Input: part model. Units: mm. Frame: model coordinates. A direction names the side the tool comes from. Round coordinates to 2 decimals unless told otherwise and drop trailing zeros. Loops run counter-clockwise (first coordinate to the right, second up) from the corner with the lowest first, then second, coordinate; pieces in that order, holes last.
1) Ray query, line 1 along Y through (x, z) = (-5, 1.45); line 2 along X through (y, z) = (-1.75, 1.5); line 3 along X through (y, z) = (4.5, 1.05). Return the intervals inside material, ascending.
2) Section D-D, the plane x = 10.5. Return loops of the section in (y, z).
3) Section C-C, the plane y = -2. Return loops of the section in (x, z), and give its area (3 significant figures).
4) Draft query along X for faces 1 (the face through (10.361, 5.245, 1.014)), 2 (the face through (0, 3, 0)), 3 (the face through (0, 2.25, 1)), 4 (the face through (-7.25, -0.05, 0.99)). Return one class per face: pulls with the +X half, pulls with the -X half, needs draft (parallel to the pull), parting line crosses it, or undercut.
5) Access query for faces 5 (the face through (-4, 7.5, 1)), 6 (the face through (7.25, 0.05, 0.99)). Directions: +Z, -Z, +X, -X, +Y, -Y. A direction counts if a zero-diameter tool reaches every point of the face in a straight line with its end or side. Return the directions, or none.
6) Section B-B, the plane x = -6.5. Return loops of the section in (y, z).
Autodesk Inventor part; units mm, degrees
ref_plane "YZ Plane" through (0, 0, 0) normal (1, 0, 0) x (0, 1, 0)
ref_plane "XZ Plane" through (0, 0, 0) normal (0, 1, 0) x (-1, 0, 0)
ref_plane "XY Plane" through (0, 0, 0) normal (0, 0, 1) x (1, 0, 0)
sketch "Skizze1" plane through (0, 0, 0) normal (0, 0, 1) x (1, 0, 0)
  line L0 (-17.5, 0) -> (17.5, 0)
  line L1 (0, -10.5) -> (0, 10.5)
  line L2 (12.5, -7.5) -> (-12.5, -7.5)
  line L3 (-12.5, -7.5) -> (-12.5, 7.5)
  line L4 (-12.5, 7.5) -> (12.5, 7.5)
  line L5 (12.5, 7.5) -> (12.5, -7.5)
  line L6 (12.5, -7.5) -> (-12.5, 7.5) construction
  line L7 (-12.5, -7.5) -> (12.5, 7.5) construction
  point P0 (0, 0)
  dimension "d0" = 15
  dimension "d1" = 25
extrude "Extrusion1" add sketch "Skizze1" along normal blind 2
fillet "Rundung1" radius 7.5 2 edges at (12.5, -7.5, 1) (12.5, 7.5, 1)
sketch "Skizze2" plane through (0, 0, 0) normal (0, 0, -1) x (-1, 0, 0)
  line L0 (17.5, 0) -> (-17.5, 0)
  line L1 (0, -10.5) -> (0, 10.5)
  line L2 (5, 0) -> (-5, 0) construction
  line L3 (5, 2.25) -> (-5, 2.25)
  line L4 (-5, -2.25) -> (5, -2.25)
  arc A0 (5, -2.25) -> (5, 2.25) centre (5, 0) ccw
  arc A1 (-5, 2.25) -> (-5, -2.25) centre (-5, 0) ccw
  point P0 (0, 0)
  dimension "d5" = 4.5
  dimension "d6" = 10
extrude "Extrusion2" cut sketch "Skizze2" against normal through all
properties part number "24_0497_0019"
Final values:
1. line 1: y = -7.5 to -2.25, 2.25 to 7.5
1. line 2: x = -12.5 to -6.41, 6.41 to 12.29
1. line 3: x = -12.5 to 11
2. outline: (-5.1, 0) - (5.1, 0) - (5.1, 2) - (-5.1, 2) - close
3. outline: (-12.5, 0) - (-6.03, 0) - (-6.03, 2) - (-12.5, 2) - close; (6.03, 0) - (12.23, 0) - (12.23, 2) - (6.03, 2) - close
3. area: 25.3 mm2
4. face 1: pulls with the +X half
4. face 2: needs draft
4. face 3: undercut
4. face 4: undercut
5. face 5: +Z, -Z, +X, -X, +Y
5. face 6: +Z, -Z
6. outline: (-7.5, 0) - (-1.68, 0) - (-1.68, 2) - (-7.5, 2) - close; (1.68, 0) - (7.5, 0) - (7.5, 2) - (1.68, 2) - close
